The drawing under review shows one solid part. Ordinate dimensions are in mm from its lowest x, y, z. A direction names the side the tool comes from. Coordinates: 2 decimals unless noted, no trailing zeros. One line per item, written item: value. Start each with the question number.
1) For pin 1 Ø6 at (x, z) = (89.41, 92.08) entering from -Y (1 decimal); pin 2 Ø8 at (y, z) = (12.7, 133.35) entering from +X (1 decimal), all flat-tipped, find the tip position at first contact; note any pin that passes through.
2) Mouldability with a two-part tool opening along X and no side actions: class the marked faces 3, 4 and 5 as released by +X, released by -X, zero draft, split by the parting line, or undercut.
3) Machinability: for the marked faces 1 and 2, which of the approach directions +Z, -Z, +X, -X, +Y, -Y give a long, thin tool a straight path to every point of the face, cutting with its end or side? Answer none if there is none.
4) For probe 1 along Z at (x, y) = (122, 12) (1 decimal); probe 2 along Y at (x, z) = (20.5, 78) (1 decimal), list the stretches that pass through material, from the lowest coordinate up. Write a range as from..to.
5) Add section B-B (z = 102.5). State how many separate pieces and enclosed holes the cut face has.
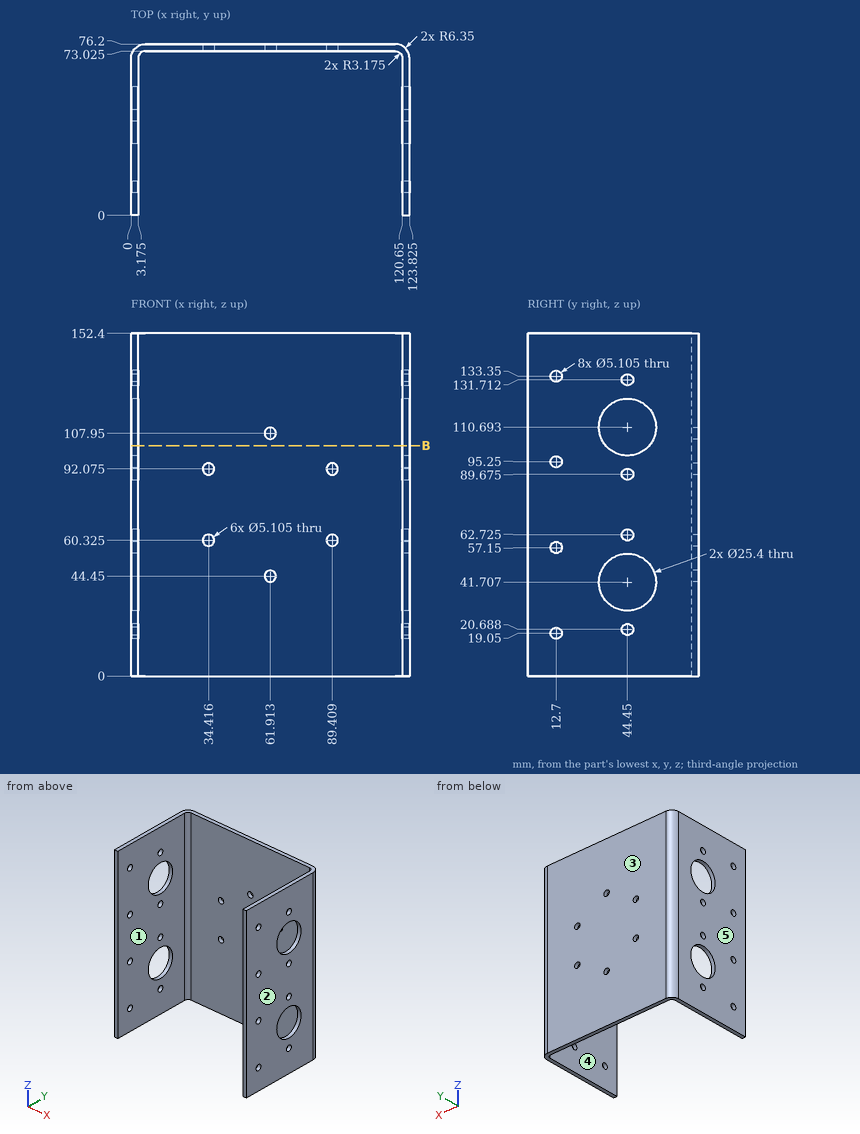
Numbers:
1. pin 1: y = 73
1. pin 2: x = 123.8
2. face 3: zero draft
2. face 4: undercut
2. face 5: released by -X
3. face 1: +Z, -Z, -Y
3. face 2: +Z, -Z, +X, +Y, -Y
4. probe 1: 0..16.6, 21.5..54.7, 59.6..92.8, 97.7..130.9, 135.8..152.4
4. probe 2: 73..76.2
5. separate pieces: 3
5. enclosed holes: 0
